CAD build for the part. Positions are in the model's coordinates, mm. Round coordinates to 2 decimals unless told otherwise and drop trailing zeros. Write each loop counter-clockwise with the first axis right and the second up, starting at its lowest first coordinate (ties: lowest second). Pieces come first, ordered by that corner, then holes. Notation, with made-up numbers: (-17.75, 27) - (30.25, 27) arc R18 cw to (30.25, 60) - close; hole circle Ø8 at (10, 86). An arc over 180 degrees is marked (long way). Answer in a Markdown table with one row per item.
```python
from build123d import *

# Parameters (mm, degrees)
SKETCH1_W                                       = 650
SKETCH1_H                                       = 270
BOSS_EXTRUDE1_DEPTH                             = 6
SKETCH2_W                                       = 35
SKETCH2_H                                       = 45
CUT_EXTRUDE1_DEPTH                              = 358.995810031
CSK_FOR_M4_FLAT_HEAD_MACHINE_SCREW1_D           = 4.2
CSK_FOR_M4_FLAT_HEAD_MACHINE_SCREW1_CSINK_D     = 8
CSK_FOR_M4_FLAT_HEAD_MACHINE_SCREW1_CSINK_ANGLE = 90


with BuildPart() as part:
    # Sketch1 → Boss-Extrude1 (new body)
    with BuildSketch(Plane(origin=(0, 0, 0), x_dir=(1, 0, 0), z_dir=(0, 1, 0))):
        with Locations((0, -15)):
            Rectangle(SKETCH1_W, SKETCH1_H)
    extrude(amount=BOSS_EXTRUDE1_DEPTH)

    # Sketch2 → Cut-Extrude1 (cut, through all)
    with BuildSketch(Plane(origin=(0, 6, 0), x_dir=(1, 0, 0), z_dir=(0, 1, 0))):
        with Locations((307.5, -127.5)):
            Rectangle(SKETCH2_W, SKETCH2_H)
        Polygon((337.933434696, -105), (325, -105), (325, -150), (290, -150), (290, -185.199938578), (337.933434696, -185.199938578), align=None)
    extrude(amount=-CUT_EXTRUDE1_DEPTH, mode=Mode.SUBTRACT)

    # CSK for M4 Flat Head Machine Screw1 (through all)
    with Locations(Plane(origin=(0, 6, 0), x_dir=(1, 0, 0), z_dir=(0, 1, 0))):
        with Locations((-310, 0), (-5, 105), (314, -39)):
            CounterSinkHole(CSK_FOR_M4_FLAT_HEAD_MACHINE_SCREW1_D / 2, CSK_FOR_M4_FLAT_HEAD_MACHINE_SCREW1_CSINK_D / 2, counter_sink_angle=CSK_FOR_M4_FLAT_HEAD_MACHINE_SCREW1_CSINK_ANGLE)


solid = part.part
```
Q1. Saw through at A-A on z = 129.5. List the corners of the cut face in (x, y).
Computed:
| item | result |
|---|---|
| outline | (-325, 0) - (290, 0) - (290, 6) - (-325, 6) - close |
Q2. Drill centre lines: line 1 (Z direction, x = -5, y = 0.95); line 2 (Z direction, x = 314, y = 1.3); line 3 (X direction, y = 2.3, z = 39). Where is each one in solid material? Low to high.
Computed:
| item | result |
|---|---|
| line 1 | z = -120 to -107.1, -102.9 to 150 |
| line 2 | z = -120 to 36.9, 41.1 to 105 |
| line 3 | x = -325 to 311.9, 316.1 to 325 |
Q3. Flat gauge pin, fed straight in: pin 1 (3 mm diameter, centred on x = 310, y = 1.5, fed in from +Z). Where does the tip first touch, or does it go through?
Computed:
| item | result |
|---|---|
| pin 1 | stops at z = 105 |
